from build123d import *

# Parameters (mm, degrees)
F0_W        = 32
F0_H        = 4
F1_DEPTH    = 8
F3_DEPTH    = 4
F4_DEPTH    = 25
F5_R        = 1.5
F6_DEPTH    = 40
F7_T1_DEPTH = 29
F7_T3_DEPTH = 29


# Not quite as in the source:
# - a fillet or chamfer that OpenCascade refuses, or shapes differently, is made with other operations: its cross-section is extruded or revolved along the edge and cut away or added


with BuildPart() as f1:
    # F0 (on Top) → F1 (new body)
    with BuildSketch(Plane.XY):
        with Locations((-2, 13.5)):
            Rectangle(F0_W, F0_H)
        Polygon((14, 11.5), (14, -11.5), (14, -15.5), (18, -15.5), (18, 0), (18, 15.5), (14, 15.5), align=None)
        with Locations((-2, -13.5)):
            Rectangle(F0_W, F0_H)
    extrude(amount=F1_DEPTH)

    # F2 (on face) → F3 (join, through all)
    with BuildSketch(Plane.YZ.offset(18)):
        with BuildLine():
            Line((-15.4216540828, 12.0949916113), (-15.5, 8))
            Line((-15.5, 8), (-6.25, 8))
            ThreePointArc((-6.25, 8), (-6.4923756022, 9.6147401314), (-7.1981402517, 11.0871625858))
            ThreePointArc((-7.1981402517, 11.0871625858), (-8.3515353126, 12.3244002785), (-9.8263607896, 13.1526315789))
            ThreePointArc((-9.8263607896, 13.1526315789), (-11.75, 11.7), (-13.6736392104, 13.1526315789))
            ThreePointArc((-13.6736392104, 13.1526315789), (-14.5971876184, 12.7056904558), (-15.4216540828, 12.0949916113))
        make_face()
        with BuildLine():
            Line((6.25, 8), (11.75, 8))
            Line((11.75, 8), (15.5, 8))
            Line((15.5, 8), (15.4216540828, 12.0949916113))
            ThreePointArc((15.4216540828, 12.0949916113), (14.5971876184, 12.7056904558), (13.6736392104, 13.1526315789))
            ThreePointArc((13.6736392104, 13.1526315789), (11.75, 11.7), (9.8263607896, 13.1526315789))
            ThreePointArc((9.8263607896, 13.1526315789), (8.3515353126, 12.3244002785), (7.1981402517, 11.0871625858))
            ThreePointArc((7.1981402517, 11.0871625858), (6.4923756022, 9.6147401314), (6.25, 8))
        make_face()
        with BuildLine():
            Line((-14.1999293119, 18.7123082578), (-15.4216540828, 12.0949916113))
            ThreePointArc((-15.4216540828, 12.0949916113), (-14.5971876184, 12.7056904558), (-13.6736392104, 13.1526315789))
            ThreePointArc((-13.6736392104, 13.1526315789), (-12.0263345611, 15.6808178135), (-9.75, 13.7))
            ThreePointArc((-9.75, 13.7), (-9.7525078538, 13.5998744499), (-9.7600251258, 13.5))
            Line((-9.7600251258, 13.5), (-7.7054746686, 13.5))
            Line((-7.7054746686, 13.5), (-8.8014388457, 18.7123082578))
            Line((-8.8014388457, 18.7123082578), (-14.1999293119, 18.7123082578))
        make_face()
        with BuildLine():
            ThreePointArc((-9.8263607896, 13.1526315789), (-8.3515353126, 12.3244002785), (-7.1981402517, 11.0871625858))
            Line((-7.1981402517, 11.0871625858), (-7.7054746686, 13.5))
            Line((-7.7054746686, 13.5), (-9.7600251258, 13.5))
            ThreePointArc((-9.7600251258, 13.5), (-9.7855000622, 13.3248467056), (-9.8263607896, 13.1526315789))
        make_face()
        with BuildLine():
            ThreePointArc((13.6736392104, 13.1526315789), (14.5971876184, 12.7056904558), (15.4216540828, 12.0949916113))
            Line((15.4216540828, 12.0949916113), (14.1999293119, 18.7123082578))
            Line((14.1999293119, 18.7123082578), (8.8014388457, 18.7123082578))
            Line((8.8014388457, 18.7123082578), (7.7054746686, 13.5))
            Line((7.7054746686, 13.5), (9.7600251258, 13.5))
            ThreePointArc((9.7600251258, 13.5), (11.6498744499, 15.6974921462), (13.75, 13.7))
            ThreePointArc((13.75, 13.7), (13.7308178135, 13.4236654389), (13.6736392104, 13.1526315789))
        make_face()
        with BuildLine():
            Line((7.7054746686, 13.5), (7.1981402517, 11.0871625858))
            ThreePointArc((7.1981402517, 11.0871625858), (8.3515353126, 12.3244002785), (9.8263607896, 13.1526315789))
            ThreePointArc((9.8263607896, 13.1526315789), (9.7855000622, 13.3248467056), (9.7600251258, 13.5))
            Line((9.7600251258, 13.5), (7.7054746686, 13.5))
        make_face()
    extrude(amount=-F3_DEPTH)

    # F2 (on face) → F4 (cut)
    with BuildSketch(Plane.YZ.offset(18)):
        with BuildLine():
            ThreePointArc((9.7600251258, 13.5), (9.7855000622, 13.3248467056), (9.8263607896, 13.1526315789))
            ThreePointArc((9.8263607896, 13.1526315789), (10.7726243517, 13.4124612555), (11.75, 13.5))
            Line((11.75, 13.5), (9.7600251258, 13.5))
        make_face()
        with BuildLine():
            ThreePointArc((11.75, 13.5), (10.7726243517, 13.4124612555), (9.8263607896, 13.1526315789))
            ThreePointArc((9.8263607896, 13.1526315789), (11.75, 11.7), (13.6736392104, 13.1526315789))
            ThreePointArc((13.6736392104, 13.1526315789), (12.7273756483, 13.4124612555), (11.75, 13.5))
        make_face()
        with BuildLine():
            ThreePointArc((11.75, 13.5), (12.7273756483, 13.4124612555), (13.6736392104, 13.1526315789))
            ThreePointArc((13.6736392104, 13.1526315789), (13.7308178135, 13.4236654389), (13.75, 13.7))
            ThreePointArc((13.75, 13.7), (11.6498744499, 15.6974921462), (9.7600251258, 13.5))
            Line((9.7600251258, 13.5), (11.75, 13.5))
        make_face()
        with BuildLine():
            ThreePointArc((-11.75, 13.5), (-12.7273756483, 13.4124612555), (-13.6736392104, 13.1526315789))
            ThreePointArc((-13.6736392104, 13.1526315789), (-11.75, 11.7), (-9.8263607896, 13.1526315789))
            ThreePointArc((-9.8263607896, 13.1526315789), (-10.7726243517, 13.4124612555), (-11.75, 13.5))
        make_face()
        with BuildLine():
            ThreePointArc((-11.75, 13.5), (-10.7726243517, 13.4124612555), (-9.8263607896, 13.1526315789))
            ThreePointArc((-9.8263607896, 13.1526315789), (-9.7855000622, 13.3248467056), (-9.7600251258, 13.5))
            Line((-9.7600251258, 13.5), (-11.75, 13.5))
        make_face()
        with BuildLine():
            ThreePointArc((-9.75, 13.7), (-12.0263345611, 15.6808178135), (-13.6736392104, 13.1526315789))
            ThreePointArc((-13.6736392104, 13.1526315789), (-12.7273756483, 13.4124612555), (-11.75, 13.5))
            Line((-11.75, 13.5), (-9.7600251258, 13.5))
            ThreePointArc((-9.7600251258, 13.5), (-9.7525078538, 13.5998744499), (-9.75, 13.7))
        make_face()
    extrude(amount=-F4_DEPTH, mode=Mode.SUBTRACT)

    # F5 (on face) → F6 (cut)
    with BuildSketch(Plane.XZ.offset(15.5)):
        with Locations((-12, 4)):
            Circle(F5_R)
        with Locations((3, 4)):
            Circle(F5_R)
    extrude(amount=-F6_DEPTH, mode=Mode.SUBTRACT)

    # F7: fillet of radius 5 on 4 edges, made by hand

    # F7_s2 → F7_t1 (cut)
    with BuildSketch(Plane.XZ.offset(-1)):
        with BuildLine():
            ThreePointArc((-18, 3), (-16.5355339059, 6.5355339059), (-13, 8))
            Line((-13, 8), (-18, 8))
            Line((-18, 8), (-18, 3))
        make_face()
        with BuildLine():
            ThreePointArc((-13, 0), (-16.5355339059, 1.4644660941), (-18, 5))
            Line((-18, 5), (-18, 0))
            Line((-18, 0), (-13, 0))
        make_face()
    extrude(amount=F7_T1_DEPTH, mode=Mode.SUBTRACT)

    # F7_s4 → F7_t3 (cut)
    with BuildSketch(Plane.XZ.offset(-28)):
        with BuildLine():
            ThreePointArc((-18, 3), (-16.5355339059, 6.5355339059), (-13, 8))
            Line((-13, 8), (-18, 8))
            Line((-18, 8), (-18, 3))
        make_face()
        with BuildLine():
            ThreePointArc((-18, 5), (-16.5355339059, 1.4644660941), (-13, 0))
            Line((-13, 0), (-18, 0))
            Line((-18, 0), (-18, 5))
        make_face()
    extrude(amount=F7_T3_DEPTH, mode=Mode.SUBTRACT)


solid = f1.part
Design review of the part built by this model. Coordinates are the model's own, in mm. A direction names the side the tool comes from. Coordinates: 2 decimals unless noted, no trailing zeros. Write each loop counter-clockwise with the first axis right and the second up, starting at its lowest first coordinate (ties: lowest second). Pieces come first, ordered by that corner, then holes. Notation, with made-up numbers: (-38.75, 22.5) -> (20.25, 22.5) arc R11 ccw to (20.25, 41.5) -> close; hole circle Ø3 at (6, 65.5). An arc over 180 degrees is marked (long way). Write each question's results on one line, items separated by ' | '. Start each with the question number.
(1) For line 1 along Z through (x, y) = (3, 13); line 2 along Y through (x, z) = (10, 7.25); line 3 along X through (y, z) = (13, 3.25), list the stretches that pass through material, from the lowest coordinate up. Write a range as from..to.
(2) The part is to be moulded in two halves that separate along Y. For faces 6 (the face through (0, 14, 8)), 7 (the face through (16.028, -14.802, 15.45)), 8 (the face through (16.028, -6.486, 9.593)), say which applies: pulls with the +Y half, pulls with the -Y half, needs draft (parallel to the pull), parting line crosses it, or undercut.
(3) Take a section at A-A on x = -1. Write out the cut boundary in (y, z).
(4) Clearance check with flat-ended pins moving along their axes: P1, Ø2.5, axis at x = -12, z = 4, coming from the -Y side; P2, Ø2, axis at x = 16, y = -2, coming from the +Z side. State where each tip first meets the part, or that it passes through.
(5) Take a section at C-C on y = -10.5. Write out the cut boundary in (x, z), and give its area (3 significant figures).
(6) Take a section at D-D on z = 6. Write out the cut boundary in (x, y), and give its area (3 significant figures).
(7) Tool access review of faces 1 (the face through (16, 0, 8)), 2 (the face through (-2, -11.5, 4)), 3 (the face through (14, 0, 7)), 4 (the face through (-13.5, -13.53, 4.07)), 5 (the face through (0, -13, 8)): name each direction out of +Z, -Z, +X, -X, +Y, -Y from which nothing blocks a thin tool from reaching the whole face with its end or side.
(8) Take a section at B-B on x = -12. Write out the cut boundary in (y, z).
Results found:
1) line 1: z = 0..2.5, 5.5..8 | line 2: y = -15.5..-11.5, 11.5..15.5 | line 3: x = -17.68..-13.3, -10.7..1.7, 4.3..18
2) face 6: needs draft | face 7: pulls with the -Y half | face 8: undercut
3) outline: (-15.5, 0) -> (-11.5, 0) -> (-11.5, 8) -> (-15.5, 8) -> close; (11.5, 0) -> (15.5, 0) -> (15.5, 8) -> (11.5, 8) -> close
4) P1: passes through | P2: stops at z = 8
5) outline: (14, 0) -> (18, 0) -> (18, 12.14) -> (14, 12.14) -> close; (14, 15.26) -> (18, 15.26) -> (18, 18.71) -> (14, 18.71) -> close | area: 62.4 mm2
6) outline: (-17, -15.5) -> (18, -15.5) -> (18, 15.5) -> (-17, 15.5) -> (-17, 11.5) -> (14, 11.5) -> (14, -11.5) -> (-17, -11.5) -> close | area: 372 mm2
7) face 1: +Z, +X, -X | face 2: +Z, -Z, -X | face 3: +Z, -X | face 4: +Y, -Y | face 5: +Z, -X, +Y, -Y
8) outline: (-15.5, 0) -> (-11.5, 0) -> (-11.5, 2.5) -> (-15.5, 2.5) -> close; (-15.5, 5.5) -> (-11.5, 5.5) -> (-11.5, 8) -> (-15.5, 8) -> close; (11.5, 0) -> (15.5, 0) -> (15.5, 2.5) -> (11.5, 2.5) -> close; (11.5, 5.5) -> (15.5, 5.5) -> (15.5, 8) -> (11.5, 8) -> close
